The model under review builds one solid part; all positions refer to its coordinate system, in mm. Face numbers are marked on the shaded views. A direction names the side the tool comes from. Round coordinates to 2 decimals unless told otherwise and drop trailing zeros. Write each loop counter-clockwise with the first axis right and the second up, starting at its lowest first coordinate (ties: lowest second). Pieces come first, ordered by that corner, then holes. Notation, with made-up numbers: (17.5, -4) - (59.5, -4) arc R18 ccw to (59.5, 27) - close; hole circle Ø3 at (-32.5, 70.25). An arc over 180 degrees is marked (long way). Write each question's results on one line, items separated by ' | '.
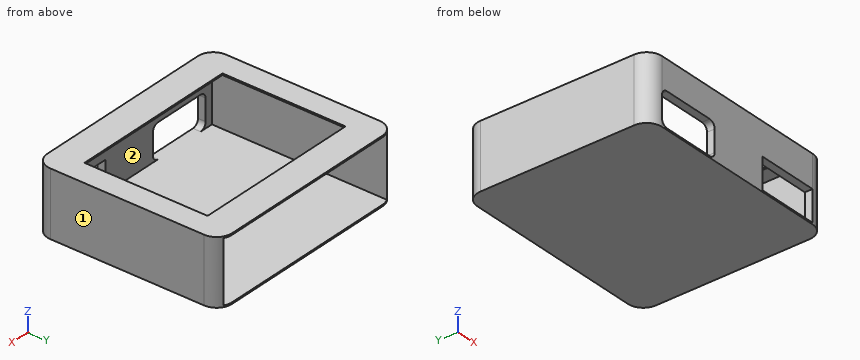
```python
from build123d import *

# Parameters (mm, degrees)
F0_W      = 70
F0_H      = 60
F1_DEPTH  = 21
F2_R      = 5
F3_W      = 65
F3_H      = 20
F4_DEPTH  = 57.5
F5_W      = 55
F5_H      = 40
F6_DEPTH  = 1
F8_DEPTH  = 5
F9_W      = 20
F9_H      = 10
F10_DEPTH = 4


with BuildPart() as f1:
    # F0 (on Top) → F1 (new body)
    with BuildSketch(Plane.XY):
        Rectangle(F0_W, F0_H)
    extrude(amount=F1_DEPTH)

    # F2
    f2_edges = [f1.edges().sort_by_distance(p)[0] for p in [
        (-35, -30, 10.5),
        (-35, 30, 10.5),
        (35, 30, 10.5),
        (35, -30, 10.5),
    ]]
    fillet(f2_edges, radius=F2_R)

    # F3 (on face) → F4 (cut)
    with BuildSketch(Plane(origin=(0, 30, 0), x_dir=(-1, 0, 0), z_dir=(0, 1, 0))):
        with Locations((0, 10.5)):
            Rectangle(F3_W, F3_H)
    extrude(amount=-F4_DEPTH, mode=Mode.SUBTRACT)

    # F5 (on face) → F6 (cut)
    with BuildSketch(Plane.XY.offset(21)):
        Rectangle(F5_W, F5_H)
    extrude(amount=-F6_DEPTH, mode=Mode.SUBTRACT)

    # F7 (on face) → F8 (cut)
    with BuildSketch(Plane.XZ.offset(30)):
        with BuildLine():
            ThreePointArc((-9, 9.5), (-9.585786, 10.914214), (-11, 11.5))
            Line((-11, 11.5), (-28, 11.5))
            ThreePointArc((-28, 11.5), (-29.414214, 10.914214), (-30, 9.5))
            Line((-30, 9.5), (-30, 2.5))
            ThreePointArc((-30, 2.5), (-29.414214, 1.085786), (-28, 0.5))
            Line((-28, 0.5), (-11, 0.5))
            ThreePointArc((-11, 0.5), (-9.585786, 1.085786), (-9, 2.5))
            Line((-9, 2.5), (-9, 9.5))
        make_face()
    extrude(amount=-F8_DEPTH, mode=Mode.SUBTRACT)

    # F9 (on face) → F10 (cut)
    with BuildSketch(Plane.XZ.offset(30)):
        with Locations((20, 5.5)):
            Rectangle(F9_W, F9_H)
    extrude(amount=-F10_DEPTH, mode=Mode.SUBTRACT)


solid = f1.part
```
Q1. Tool access review of the marked faces 1 and 2: name each direction out of +Z, -Z, +X, -X, +Y, -Y from which nothing blocks a thin tool from reaching the whole face with its end or side.
Evaluation:
face 1: +Z, -Z, +X, +Y, -Y | face 2: +Y
Q2. We need section B-B (z = 12.5). State the section outline as (x, y) points.
Evaluation:
outline: (-35, -25) arc R5 ccw to (-30, -30) - (30, -30) arc R5 ccw to (35, -25) - (35, 25) arc R5 ccw to (32.5, 29.33) - (32.5, -27.5) - (-32.5, -27.5) - (-32.5, 29.33) arc R5 ccw to (-35, 25) - close
Q3. For probe 1 along Z at (x, y) = (-18.5, 22); probe 2 along X at (y, z) = (20, 2.5); probe 3 along Y at (x, z) = (21.5, 17.75), list the stretches that pass through material, from the lowest coordinate up.
Evaluation:
probe 1: z = 0 to 0.5, 20.5 to 21 | probe 2: x = -35 to -32.5, 32.5 to 35 | probe 3: y = -30 to -27.5
Q4. Insertion check: P1, Ø2, axis at x = 20, y = -29, coming from the -Z side; P2, Ø0.8, axis at y = -28.5, z = 7, coming from the +X side; P3, Ø2, axis at x = -19.5, z = 13, coming from the +Y side; P4, Ø3, axis at y = -29, z = 7, coming from the -X side. Each pin has a flat end and moves straight along its axis. Give the tip position at first contact, or say it passes through.
Evaluation:
P1: stops at z = 0 | P2: stops at x = 33.92 | P3: stops at y = -27.5 | P4: stops at x = -34.33
Q5. We need section A-A (x = -23). State the section outline as (y, z) points.
Evaluation:
outline: (-30, 0) - (30, 0) - (30, 0.5) - (-30, 0.5) - close; (-30, 11.5) - (-27.5, 11.5) - (-27.5, 20.5) - (-20, 20.5) - (-20, 21) - (-30, 21) - close; (20, 20.5) - (30, 20.5) - (30, 21) - (20, 21) - close
Q6. We need section D-D (x = -4.5). State the section outline as (y, z) points.
Evaluation:
outline: (-30, 0) - (30, 0) - (30, 0.5) - (-27.5, 0.5) - (-27.5, 20.5) - (-20, 20.5) - (-20, 21) - (-30, 21) - close; (20, 20.5) - (30, 20.5) - (30, 21) - (20, 21) - close
Q7. We need section C-C (y = -10). State the section outline as (x, z) points, plus the area to 4 significant figures.
Evaluation:
outline: (-35, 0) - (35, 0) - (35, 21) - (27.5, 21) - (27.5, 20.5) - (32.5, 20.5) - (32.5, 0.5) - (-32.5, 0.5) - (-32.5, 20.5) - (-27.5, 20.5) - (-27.5, 21) - (-35, 21) - close | area: 142.5 mm^2
